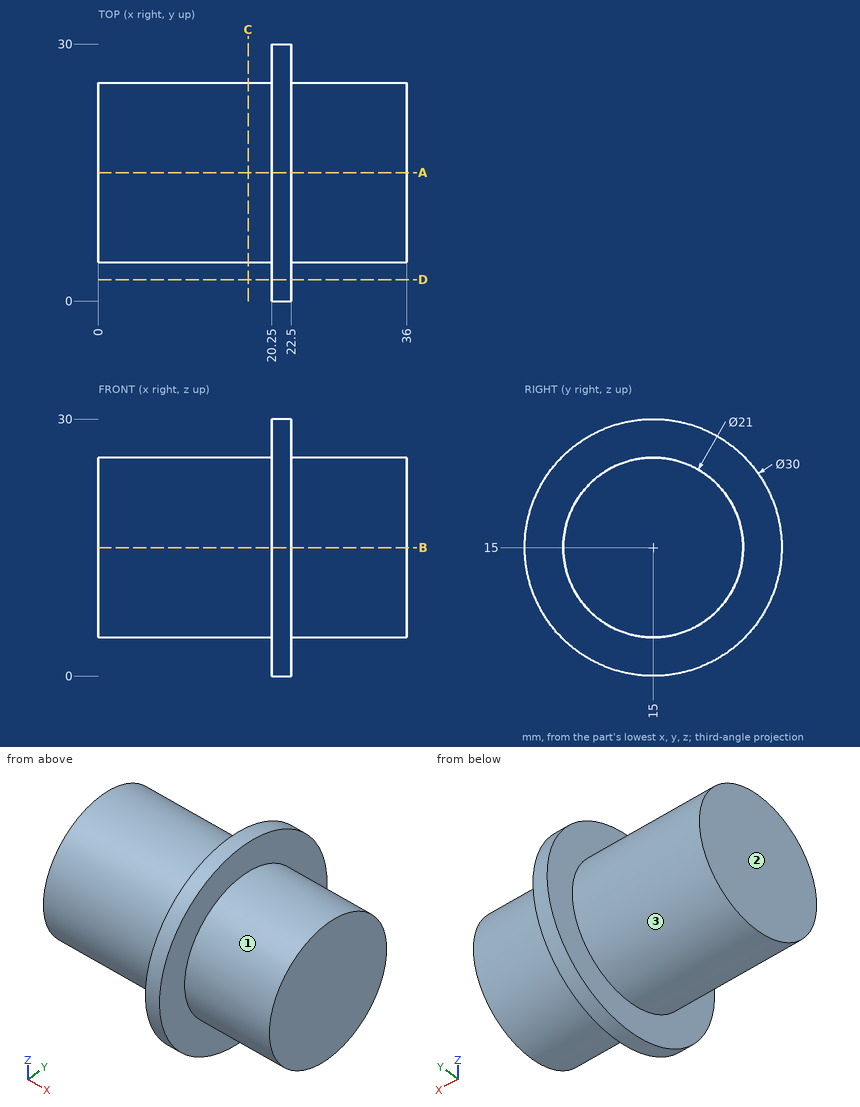
Design review of the part shown in the three views and the two pictorial views. Dimensions are in mm from the part's minimum x, y and z. A direction names the side the tool comes from. Coordinates: 2 decimals unless noted, no trailing zeros. Loops run counter-clockwise (first coordinate to the right, second up) from the corner with the lowest first, then second, coordinate; pieces in that order, holes last. Notation, with made-up numbers: (12.5, 16.25) -> (33.5, 16.25) arc R13 cw to (33.5, 32.25) -> close; hole circle Ø9 at (54.5, -20.75). An arc over 180 degrees is marked (long way). Answer as CSV lines item,"result".
Item 1: Take a section at D-D, the plane y = 2.5. State the section outline as (x, z) points.
Results below:
outline,"(20.25, 6.71) -> (22.5, 6.71) -> (22.5, 23.29) -> (20.25, 23.29) -> close"
Item 2: For L1, parallel to X at y = 18, z = 3; L2, parallel to Z at x = 15, y = 24.5, list the stretches that pass through material, from the lowest coordinate up.
Results below:
L1,"x = 20.25 to 22.5"
L2,"z = 10.53 to 19.47"
Item 3: Insertion check: pin 1 (4 mm diameter, centred on x = 15.5, y = 8.5, fed in from +Z); pin 2 (12 mm diameter, centred on x = 17.5, z = 5.5, fed in from +Y); pin 3 (1 mm diameter, centred on x = 32.5, z = 25, fed in from +Y). Each pin has a flat end and moves straight along its axis. Give the tip position at first contact, or say it passes through.
Results below:
pin 1,"stops at z = 24.49"
pin 2,"stops at y = 29.41"
pin 3,"stops at y = 19.47"
Item 4: Machinability: for the marked faces 1, 2 and 3, which of the approach directions +Z, -Z, +X, -X, +Y, -Y give a long, thin tool a straight path to every point of the face, cutting with its end or side? Answer none if there is none.
Results below:
face 1,"+X"
face 2,"+Z, -Z, -X, +Y, -Y"
face 3,"-X"
Item 5: Take a section at A-A, the plane y = 15. State the section outline as (x, z) points.
Results below:
outline,"(0, 4.5) -> (20.25, 4.5) -> (20.25, 0) -> (22.5, 0) -> (22.5, 4.5) -> (36, 4.5) -> (36, 25.5) -> (22.5, 25.5) -> (22.5, 30) -> (20.25, 30) -> (20.25, 25.5) -> (0, 25.5) -> close"
Item 6: Take a section at C-C, the plane x = 17.5. State the section outline as (y, z) points.
Results below:
outline,"circle Ø21 at (15, 15)"
